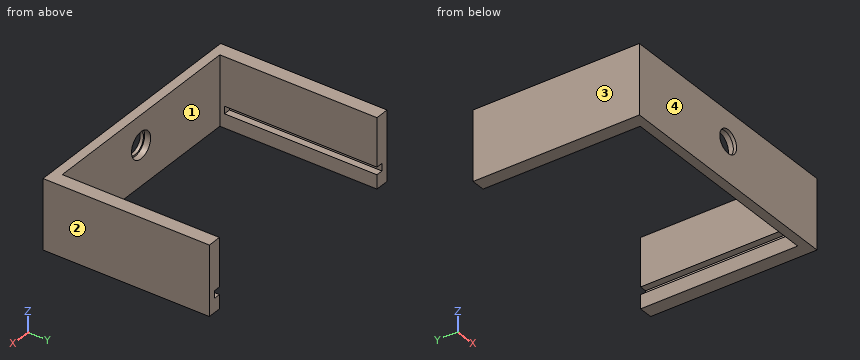
from build123d import *

# Parameters (mm, degrees)
BOX004_W               = 50
BOX004_H               = 33
BOX004_DEPTH           = 1.6
BOX002_W               = 3
BOX002_H               = 36
BOX002_DEPTH           = 15
BOX001_W               = 3
BOX001_H               = 36
BOX001_DEPTH           = 15
CYLINDER001_R          = 2.85
CYLINDER001_DEPTH      = 1.3
CYLINDER001_ROLL_ANGLE = 90
CYLINDER_R             = 2.5
CYLINDER_DEPTH         = 0.7
CYLINDER_ROLL_ANGLE    = 90
BOX003_W               = 53
BOX003_H               = 2
BOX003_DEPTH           = 15


with BuildPart() as pcb:
    # Box004 → Box004 (new body)
    with BuildSketch(Plane(origin=(1.5, 3, 3), x_dir=(1, 0, 0), z_dir=(0, 0, 1))):
        with Locations((25, 16.5)):
            Rectangle(BOX004_W, BOX004_H)
    extrude(amount=BOX004_DEPTH)


with BuildPart() as side2:
    # Box002 → Box002 (new body)
    with BuildSketch(Plane(origin=(50, 0, 0), x_dir=(1, 0, 0), z_dir=(0, 0, 1))):
        with Locations((1.5, 18)):
            Rectangle(BOX002_W, BOX002_H)
    extrude(amount=BOX002_DEPTH)


with BuildPart() as side1:
    # Box001 → Box001 (new body)
    with BuildSketch(Plane.XY):
        with Locations((1.5, 18)):
            Rectangle(BOX001_W, BOX001_H)
    extrude(amount=BOX001_DEPTH)


with BuildPart() as cylinder001:
    # Cylinder001 → Cylinder001 (new body)
    with BuildSketch(Plane.XY):
        Circle(CYLINDER001_R)
    extrude(amount=CYLINDER001_DEPTH)


with BuildPart() as cylinder001_1:
    # Cylinder001 roll: moved
    add(cylinder001.part.rotate(Axis((0, 0, 0), (1, 0, 0)), CYLINDER001_ROLL_ANGLE))


with BuildPart() as cylinder001_2:
    # Cylinder001 placement: moved
    add(cylinder001_1.part.moved(Location((26.5, 2, 8.6))))


with BuildPart() as led:
    # Cylinder → Cylinder (new body)
    with BuildSketch(Plane.XY):
        Circle(CYLINDER_R)
    extrude(amount=CYLINDER_DEPTH)


with BuildPart() as led_1:
    # Cylinder roll: moved
    add(led.part.rotate(Axis((0, 0, 0), (1, 0, 0)), CYLINDER_ROLL_ANGLE))


with BuildPart() as led_2:
    # Cylinder placement: moved
    add(led_1.part.moved(Location((26.5, 0.7, 8.6))))

    # Fusion001: union Cylinder001
    add(cylinder001_2.part)


with BuildPart() as cut001:
    # Box003 → Box003 (new body)
    with BuildSketch(Plane.XY):
        with Locations((26.5, 1)):
            Rectangle(BOX003_W, BOX003_H)
    extrude(amount=BOX003_DEPTH)

    # Cut: cut LED
    add(led_2.part, mode=Mode.SUBTRACT)

    # Fusion: union side2, side1
    add(side2.part)
    add(side1.part)

    # Cut001: cut PCB
    add(pcb.part, mode=Mode.SUBTRACT)


solid = cut001.part
Geometry check sheet. Reference: the model listing, model coordinates, mm. Face numbers are marked on the shaded views. Round coordinates to 2 decimals unless told otherwise and drop trailing zeros. Order: outer loops, then holes, each group sorted by start corner. A loop starts at its lowest first (then second) coordinate and runs counter-clockwise, first axis right, second up. Notation, with made-up numbers: (37.25, 16) - (54.25, 16) arc R24 ccw to (54.25, 50) - close; hole circle Ø7 at (82.25, 2). An arc over 180 degrees is marked (long way). One line per question, with ' | ' between items. Start each with the question number.
(1) Depth check by flat-ended pin: pin 1 Ø6.5 at (x, z) = (25, 7.5) entering from +Y. Enter the tip coordinate at first touch or a pass-through.
(2) Release check for a two-part mould opening along X. For the marked faces 1, 2, 3 and 4 record: released by +X, released by -X, zero draft, split by the parting line, or undercut.
(3) Sectioned sample at B-B on x = 26.5. Record the cut outline in (y, z).
(4) Sectioned sample at A-A on y = 27. Record the cut outline in (x, z), and give its area (3 significant figures).
(5) Sectioned sample at D-D on z = 1.25. Record the cut outline in (x, y).
(6) Sectioned sample at C-C on z = 8.6. Record the cut outline in (x, y).
(7) Thickness scan on L1, parallel to X at y = 20.5, z = 4; L2, parallel to X at y = 12, z = 8; L3, parallel to Z at x = 26.5, y = 0.2. Record the ranges inside material, lowest first. Write a range as [from, to].
Conclusion:
1) pin 1: stops at y = 2
2) face 1: undercut | face 2: released by +X | face 3: released by -X | face 4: zero draft
3) outline: (0, 0) - (2, 0) - (2, 5.75) - (0.7, 5.75) - (0.7, 6.1) - (0, 6.1) - close; (0, 11.1) - (0.7, 11.1) - (0.7, 11.45) - (2, 11.45) - (2, 15) - (0, 15) - close
4) outline: (0, 0) - (3, 0) - (3, 3) - (1.5, 3) - (1.5, 4.6) - (3, 4.6) - (3, 15) - (0, 15) - close; (50, 0) - (53, 0) - (53, 15) - (50, 15) - (50, 4.6) - (51.5, 4.6) - (51.5, 3) - (50, 3) - close | area: 85.2 mm2
5) outline: (0, 0) - (53, 0) - (53, 36) - (50, 36) - (50, 2) - (3, 2) - (3, 36) - (0, 36) - close
6) outline: (0, 0) - (24, 0) - (24, 0.7) - (23.65, 0.7) - (23.65, 2) - (3, 2) - (3, 36) - (0, 36) - close; (29, 0) - (53, 0) - (53, 36) - (50, 36) - (50, 2) - (29.35, 2) - (29.35, 0.7) - (29, 0.7) - close
7) L1: x = [0, 1.5], [51.5, 53] | L2: x = [0, 3], [50, 53] | L3: z = [0, 6.1], [11.1, 15]
